The model under review builds one solid part; all positions refer to its coordinate system, in mm. Give positions to 0.01 mm unless a question says otherwise; leave off trailing zeros. Order: outer loops, then holes, each group sorted by start corner. A loop starts at its lowest first (then second) coordinate and runs counter-clockwise, first axis right, second up. Notation, with made-up numbers: (65.5, -15) - (76.5, -15) arc R17 ccw to (76.5, 14) - close; hole circle Ø11 at (47, -27). An arc over 180 degrees is marked (long way). Use CSV: the item, a comma, the result in double quotes. Start each with the question number.
1. Take a section at B-B, the plane y = 150. State the section outline as (x, z) points.
2. Take a section at C-C, the plane x = 0. State the section outline as (y, z) points.
3. To check wall thickness, follow line 1 (Z direction, x = -0.25, y = 150); line 2 (Y direction, x = 2.25, z = 0); line 3 (Y direction, x = 0, z = -0.5). State the ranges of each line that lie inside material, in increasing order. Write a range as [from, to].
4. Take a section at A-A, the plane z = 0. State the section outline as (x, y) points.
```python
from build123d import *

# Parameters (mm, degrees)
SKETCH1_W           = 10
SKETCH1_H           = 10
BOSS_EXTRUDE1_DEPTH = 300
SKETCH3_R           = 2.5
CUT_EXTRUDE1_DEPTH  = 301.208261046
SKETCH4_W           = 10
SKETCH4_H           = 10
CUT_EXTRUDE2_DEPTH  = 70
SKETCH5_R           = 2.5
CUT_EXTRUDE3_DEPTH  = 231.271578793


with BuildPart() as part:
    # Sketch1 → Boss-Extrude1 (new body)
    with BuildSketch(Plane(origin=(0, 0, 0), x_dir=(1, 0, 0), z_dir=(0, 1, 0))):
        Rectangle(SKETCH1_W, SKETCH1_H)
    extrude(amount=BOSS_EXTRUDE1_DEPTH)

    # Sketch3 → Cut-Extrude1 (cut, through all)
    with BuildSketch(Plane.ZY.offset(5)):
        with Locations((0, 150)):
            Circle(SKETCH3_R)
    extrude(amount=-CUT_EXTRUDE1_DEPTH, mode=Mode.SUBTRACT)

    # Sketch4 → Cut-Extrude2 (cut)
    with BuildSketch(Plane(origin=(0, 300, 0), x_dir=(1, 0, 0), z_dir=(0, 1, 0))):
        Rectangle(SKETCH4_W, SKETCH4_H)
    extrude(amount=-CUT_EXTRUDE2_DEPTH, mode=Mode.SUBTRACT)

    # Sketch5 → Cut-Extrude3 (cut, through all)
    with BuildSketch(Plane(origin=(0, 0, -5), x_dir=(-1, 0, 0), z_dir=(0, 0, -1))):
        with Locations((0, 10)):
            Circle(SKETCH5_R)
    extrude(amount=-CUT_EXTRUDE3_DEPTH, mode=Mode.SUBTRACT)


solid = part.part
```
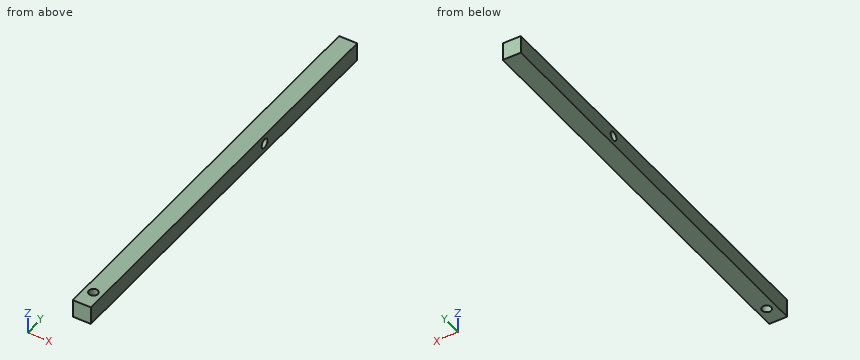
Determined:
1,outline,"(-5, -5) - (5, -5) - (5, -2.5) - (-5, -2.5) - close; (-5, 2.5) - (5, 2.5) - (5, 5) - (-5, 5) - close"
2,outline,"(0, -5) - (7.5, -5) - (7.5, 5) - (0, 5) - close; (12.5, -5) - (230, -5) - (230, 5) - (12.5, 5) - close; hole circle Ø5 at (150, 0)"
3,line 1,"z = [-5, -2.5], [2.5, 5]"
3,line 2,"y = [0, 8.91], [11.09, 147.5], [152.5, 230]"
3,line 3,"y = [0, 7.5], [12.5, 147.55], [152.45, 230]"
4,outline,"(-5, 0) - (5, 0) - (5, 147.5) - (-5, 147.5) - close; (-5, 152.5) - (5, 152.5) - (5, 230) - (-5, 230) - close; hole circle Ø5 at (0, 10)"
